from build123d import *

# Parameters (mm, degrees)
SALIENTE_EXTRUIR1_DEPTH = 6.8


with BuildPart() as part:
    # Croquis1 → Saliente-Extruir1 (new body)
    with BuildSketch(Plane(origin=(0, 0, 0), x_dir=(0, 0, -1), z_dir=(1, 0, 0))):
        with BuildLine():
            Line((65.042457404, 1.865136667), (65.16462425, 8.864070533))
            Line((65.16462425, 8.864070533), (70.163862725, 8.776808501))
            Line((70.163862725, 8.776808501), (69.989338661, -1.221668451))
            Line((69.989338661, -1.221668451), (0, -50))
            Line((0, -50), (0, 0))
            Line((0, 0), (61.9905571, -1.082049199))
            ThreePointArc((61.9905571, -1.082049199), (64.12688943, -0.240525515), (65.042457404, 1.865136667))
        make_face()
    extrude(amount=SALIENTE_EXTRUIR1_DEPTH)


solid = part.part
Here's how the part is built. I have some questions about the finished solid (model axes, mm). Coordinates: 2 decimals unless noted, no trailing zeros. Write each loop counter-clockwise with the first axis right and the second up, starting at its lowest first coordinate (ties: lowest second). Pieces come first, ordered by that corner, then holes. Notation, with made-up numbers: (-32.75, -8.5) - (4.25, -8.5) arc R28 cw to (4.25, 16.5) - close; hole circle Ø10 at (27, 47.5). An arc over 180 degrees is marked (long way). Use one line per item in the form item = value.
1) Suppose I cut it at B-B, the plane z = -21.5. Write out the boundary of the cut face in (x, y), plus the area to 3 significant figures.
Solved:
outline = (0, -35.02) - (6.8, -35.02) - (6.8, -0.38) - (0, -0.38) - close
area = 236 mm2
2) I need wall thicknesses on line 1 (Y direction, x = 1.25, z = -63); line 2 (Y direction, x = 5.25, z = -37); line 3 (Z direction, x = 1, y = 2). Which ranges of each line are inside material? Lowest first, please.
Solved:
line_1 = -6.09 to -0.93
line_2 = -24.21 to -0.65
line_3 = -70.05 to -65.04
3) Suppose I cut it at C-C, the plane y = -42. Write out the boundary of the cut face in (x, z).
Solved:
outline = (0, -11.48) - (6.8, -11.48) - (6.8, 0) - (0, 0) - close
4) Thinking about a two-plate mould opening in Z: for faces 1 (the flat face through (3, -25, 0)), 2 (the flat face through (6.8, -14, -28)), 3 (the flat face through (3.352, -25.269, -35.485)), 4 (the cylindrical face through (3.352, -0.263, -64.103)), which applies, released by +Z, released by -Z, zero draft, split by the parting line, or undercut?
Solved:
face_1 = released by +Z
face_2 = zero draft
face_3 = released by -Z
face_4 = undercut
5) Suppose I cut it at A-A, the plane x = 5. Write out the boundary of the cut face in (y, z), plus the area to 3 significant figures.
Solved:
outline = (-50, 0) - (-1.22, -69.99) - (8.78, -70.16) - (8.86, -65.16) - (1.87, -65.04) arc R3 cw to (-1.08, -61.99) - (0, 0) - close
area = 1,800 mm2
6) I'm going to push a flat-ended pin straight in: P1, Ø1.5, axis at y = -16.5, z = -43, coming from the -X side. Where does the tip first touch, or does it pass through?
Solved:
P1 = 0
